from build123d import *

# Parameters (mm, degrees)
SKETCH1_W           = 34
SKETCH1_H           = 20
BOSS_EXTRUDE1_DEPTH = 2.5
SKETCH2_R           = 3
SKETCH2_R_2         = 8.25
CUT_EXTRUDE1_DEPTH  = 5
SKETCH5_R           = 4.025
CUT_EXTRUDE4_DEPTH  = 2
SKETCH3_R           = 1.025
CUT_EXTRUDE2_DEPTH  = 4
SKETCH4_R           = 1.925
CUT_EXTRUDE3_DEPTH  = 1.5
CUT_EXTRUDE5_DEPTH  = 1.5
FILLET1_R           = 2
CHAMFER1_SIZE       = 1
FILLET2_R           = 0.3
SKETCH7_R           = 5.525
SKETCH7_R_2         = 4.025
BOSS_EXTRUDE2_DEPTH = 0.5
CUT_EXTRUDE6_DEPTH  = 1.5
SKETCH9_R           = 1.025
BOSS_EXTRUDE3_DEPTH = 0.4


with BuildPart() as part:
    # Sketch1 → Boss-Extrude1 (new body)
    with BuildSketch(Plane(origin=(0, 0, 0), x_dir=(1, 0, 0), z_dir=(0, 1, 0))):
        Rectangle(SKETCH1_W, SKETCH1_H)
    extrude(amount=BOSS_EXTRUDE1_DEPTH)

    # Sketch2 → Cut-Extrude1 (cut)
    with BuildSketch(Plane(origin=(0, 2.5, 0), x_dir=(1, 0, 0), z_dir=(0, 1, 0))):
        with Locations((-7.5, 0)):
            Circle(SKETCH2_R)
        with Locations((7.5, 0)):
            Circle(SKETCH2_R_2)
    extrude(amount=-CUT_EXTRUDE1_DEPTH, mode=Mode.SUBTRACT)

    # Sketch5 → Cut-Extrude4 (cut)
    with BuildSketch(Plane(origin=(0, 2.5, 0), x_dir=(1, 0, 0), z_dir=(0, 1, 0))):
        with Locations((-7.5, 0)):
            Circle(SKETCH5_R)
    extrude(amount=-CUT_EXTRUDE4_DEPTH, mode=Mode.SUBTRACT)

    # Sketch3 → Cut-Extrude2 (cut)
    with BuildSketch(Plane(origin=(0, 2.5, 0), x_dir=(1, 0, 0), z_dir=(0, 1, 0))):
        with Locations((15, 8)):
            Circle(SKETCH3_R)
        with Locations((-15, 8)):
            Circle(SKETCH3_R)
        with Locations((-15, -8)):
            Circle(SKETCH3_R)
        with Locations((15, -8)):
            Circle(SKETCH3_R)
    extrude(amount=-CUT_EXTRUDE2_DEPTH, mode=Mode.SUBTRACT)

    # Sketch4 → Cut-Extrude3 (cut)
    with BuildSketch(Plane(origin=(0, 2.5, 0), x_dir=(1, 0, 0), z_dir=(0, 1, 0))):
        with Locations((-15, 8)):
            Circle(SKETCH4_R)
        with Locations((-15, -8)):
            Circle(SKETCH4_R)
        with Locations((15, 8)):
            Circle(SKETCH4_R)
        with Locations((15, -8)):
            Circle(SKETCH4_R)
    extrude(amount=-CUT_EXTRUDE3_DEPTH, mode=Mode.SUBTRACT)

    # Sketch6 → Cut-Extrude5 (cut)
    with BuildSketch(Plane(origin=(0, 2.5, 0), x_dir=(1, 0, 0), z_dir=(0, 1, 0))):
        with BuildLine():
            Line((17, 10), (-17, 10))
            Line((-17, 10), (-17, 6.075))
            Line((-17, 6.075), (-15, 6.075))
            ThreePointArc((-15, 6.075), (-13.472236111, 6.828862732), (-13.141068855, 8.5))
            Line((-13.141068855, 8.5), (13.141068855, 8.5))
            ThreePointArc((13.141068855, 8.5), (13.472236111, 6.828862732), (15, 6.075))
            Line((15, 6.075), (17, 6.075))
            Line((17, 6.075), (17, 10))
        make_face()
    extrude(amount=-CUT_EXTRUDE5_DEPTH, mode=Mode.SUBTRACT)

    # Fillet1
    fillet1_edges = [part.edges().sort_by_distance(p)[0] for p in [
        (13.141068855, 1.75, -8.5),
        (-13.141068855, 1.75, -8.5),
    ]]
    fillet(fillet1_edges, radius=FILLET1_R)

    # Chamfer1
    chamfer1_edges = [part.edges().sort_by_distance(p)[0] for p in [
        (17, 1.25, 10),
        (-17, 1.25, 10),
        (-17, 0.5, -10),
        (17, 0.5, -10),
    ]]
    chamfer(chamfer1_edges, length=CHAMFER1_SIZE)

    # Fillet2
    fillet2_edges = [part.edges().sort_by_distance(p)[0] for p in [
        (0, 1, -10),
        (16.5, 1, -9.5),
        (-16.5, 1, -9.5),
    ]]
    fillet(fillet2_edges, radius=FILLET2_R)

    # Sketch7 → Boss-Extrude2 (add)
    with BuildSketch(Plane(origin=(0, 2.5, 0), x_dir=(1, 0, 0), z_dir=(0, 1, 0))):
        with Locations((-7.5, 0)):
            Circle(SKETCH7_R)
        with Locations((-7.5, 0)):
            Circle(SKETCH7_R_2, mode=Mode.SUBTRACT)
    extrude(amount=BOSS_EXTRUDE2_DEPTH)

    # Sketch8 → Cut-Extrude6 (cut)
    with BuildSketch(Plane(origin=(0, 2.5, 0), x_dir=(1, 0, 0), z_dir=(0, 1, 0))):
        with BuildLine():
            Line((-15, -6.075), (-17, -6.075))
            Line((-17, -6.075), (-17, -9))
            Line((-17, -9), (-16, -10))
            Line((-16, -10), (-13.075, -10))
            Line((-13.075, -10), (-13.075, -8))
            ThreePointArc((-13.075, -8), (-16.361180554, -9.361180554), (-15, -6.075))
        make_face()
        with BuildLine():
            Line((13.075, -10), (13.075, -8))
            ThreePointArc((13.075, -8), (16.361180554, -9.361180554), (15, -6.075))
            Line((15, -6.075), (17, -6.075))
            Line((17, -6.075), (17, -9))
            Line((17, -9), (16, -10))
            Line((16, -10), (13.075, -10))
        make_face()
    extrude(amount=-CUT_EXTRUDE6_DEPTH, mode=Mode.SUBTRACT)

    # Sketch9 → Boss-Extrude3 (add)
    with BuildSketch(Plane(origin=(0, 1, 0), x_dir=(1, 0, 0), z_dir=(0, 1, 0))):
        with BuildLine():
            Line((13.075, -8), (13.075, -10))
            Line((13.075, -10), (16, -10))
            Line((16, -10), (17, -9))
            Line((17, -9), (17, -6.075))
            Line((17, -6.075), (15, -6.075))
            ThreePointArc((15, -6.075), (13.638819446, -6.638819446), (13.075, -8))
        make_face()
        with Locations((15, -8)):
            Circle(SKETCH9_R, mode=Mode.SUBTRACT)
        with BuildLine():
            Line((-15, -6.075), (-17, -6.075))
            Line((-17, -6.075), (-17, -9))
            Line((-17, -9), (-16, -10))
            Line((-16, -10), (-13.075, -10))
            Line((-13.075, -10), (-13.075, -8))
            ThreePointArc((-13.075, -8), (-13.638819446, -6.638819446), (-15, -6.075))
        make_face()
        with Locations((-15, -8)):
            Circle(SKETCH9_R, mode=Mode.SUBTRACT)
    extrude(amount=BOSS_EXTRUDE3_DEPTH)


solid = part.part
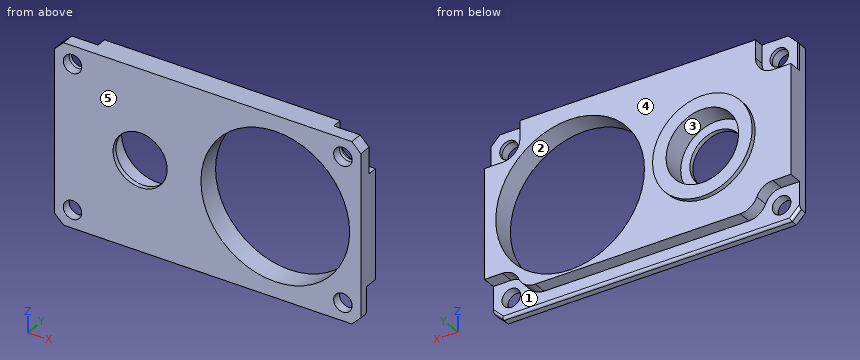
Model file for the job. Use its own axes, mm. Face numbers are marked on the shaded views. A direction names the side the tool comes from. Give positions to 0.01 mm unless a question says otherwise; leave off trailing zeros. Write each loop counter-clockwise with the first axis right and the second up, starting at its lowest first coordinate (ties: lowest second). Pieces come first, ordered by that corner, then holes. Notation, with made-up numbers: (89, 73.5) - (121, 73.5) arc R36 ccw to (121, 107.5) - close; hole circle Ø11 at (88.5, 81.5). An arc over 180 degrees is marked (long way). Answer as CSV lines item,"result".
1. Band-saw the part on C-C (y = 1.75). Write the cut outline in (x, z) (3 decimals), and give its area (3 significant figures).
Responses:
outline,"(-17, -6.075) - (-15, -6.075) arc R1.925 cw to (-13.221, -7.264) arc R2 ccw to (-11.373, -8.5) - (11.373, -8.5) arc R2 ccw to (13.221, -7.264) arc R1.925 cw to (15, -6.075) - (17, -6.075) - (17, 6.075) - (15, 6.075) arc R1.925 cw to (13.075, 8) - (13.075, 10) - (-13.075, 10) - (-13.075, 8) arc R1.925 cw to (-15, 6.075) - (-17, 6.075) - close; hole circle Ø8.05 at (-7.5, 0); hole circle Ø16.5 at (7.5, 0)"
area,"317 mm2"
2. Band-saw the part on A-A (x = 7.5). Write the cut outline in (y, z).
Responses:
outline,"(0, -10) - (0.7, -10) arc R0.3 ccw to (1, -9.7) - (1, -8.5) - (2.5, -8.5) - (2.5, -8.25) - (0, -8.25) - close; (0, 8.25) - (2.5, 8.25) - (2.5, 10) - (0, 10) - close"
3. Drill centre lines: L1, parallel to Z at x = -15, y = 0.75 (3 decimals); L2, parallel to Z at x = 7.5, y = 2; L3, parallel to X at y = 1.95, z = 0 (3 decimals). Where is each one in solid material? Low to high. Write a range as [from, to].
Responses:
L1,"z = [-9.996, -9.025], [-6.975, 6.975], [9.025, 10]"
L2,"z = [-8.5, -8.25], [8.25, 10]"
L3,"x = [-17, -11.525], [-3.475, -0.75], [15.75, 17]"
4. Band-saw the part on B-B (z = 0). Write the cut outline in (x, y) (3 decimals).
Responses:
outline,"(-17, 0) - (-10.5, 0) - (-10.5, 0.5) - (-11.525, 0.5) - (-11.525, 3) - (-13.025, 3) - (-13.025, 2.5) - (-17, 2.5) - close; (-4.5, 0) - (-0.75, 0) - (-0.75, 2.5) - (-1.975, 2.5) - (-1.975, 3) - (-3.475, 3) - (-3.475, 0.5) - (-4.5, 0.5) - close; (15.75, 0) - (17, 0) - (17, 2.5) - (15.75, 2.5) - close"
5. Pin check, flat tips, straight feed: pin 1 (1.6 mm diameter, centred on x = 16, y = 2, fed in from -Z) (3 decimals); pin 2 (1.2 mm diameter, centred on x = 15.5, z = 7.5, fed in from +Y); pin 3 (1.8 mm diameter, centred on x = 3, z = -7.5, fed in from +Y); pin 4 (3.5 mm diameter, centred on x = 15, z = -8, fed in from -Y). Stop position of each tip, or through.
Responses:
pin 1,"stops at z = -6.075"
pin 2,"stops at y = 1.4"
pin 3,"stops at y = 2.5"
pin 4,"stops at y = 0"
6. Two-plate mould, pull along X, no slides. Class the marked faces 1, 2 and 3: +X half, -X half, draft (parallel to the pull), parting line (faces both ways), or undercut.
Responses:
face 1,"draft"
face 2,"undercut"
face 3,"undercut"
7. 3-axis set-ups, long thin cutter, end or side, ignore diameter. For the marked faces 4 and 5: which of +Z, -Z, +X, -X, +Y, -Y reach the whole face in a straight line?
Responses:
face 4,"+Y"
face 5,"+Z, -Z, +X, -X, -Y"
8. Band-saw the part on D-D (z = 6.5). Write the cut outline in (x, y), and give its area (3 significant figures).
Responses:
outline,"(-17, 0) - (2.42, 0) - (2.42, 2.5) - (-13.79, 2.5) - (-13.79, 1.4) - (-17, 1.4) - close; (12.58, 0) - (17, 0) - (17, 1.4) - (13.79, 1.4) - (13.79, 2.5) - (12.58, 2.5) - close"
area,"52.5 mm2"
